```python
from build123d import *

# Parameters (mm, degrees)
IZIM2_R                     = 1
Y_KSEKLIK_EKSTR_ZYON1_DEPTH = 3


with BuildPart() as part:
    # Çizim2 → Yükseklik-Ekstrüzyon1 (new body)
    with BuildSketch(Plane(origin=(0, 0, 0), x_dir=(1, 0, 0), z_dir=(0, 1, 0))):
        with BuildLine():
            Line((2.727931774, -0.347689854), (2.491435912, -0.206753706))
            Line((2.491435912, -0.206753706), (2.246916453, -0.117755902))
            ThreePointArc((2.246916453, -0.117755902), (2.25, 0), (2.246916453, 0.117755902))
            Line((2.246916453, 0.117755902), (2.491435912, 0.206753706))
            Line((2.491435912, 0.206753706), (2.727931774, 0.347689854))
            ThreePointArc((2.727931774, 0.347689854), (2.716142937, 0.430194779), (2.701859364, 0.512304577))
            Line((2.701859364, 0.512304577), (2.433386768, 0.573261578))
            Line((2.433386768, 0.573261578), (2.173333109, 0.582342851))
            ThreePointArc((2.173333109, 0.582342851), (2.139877162, 0.695288237), (2.10055596, 0.806327886))
            Line((2.10055596, 0.806327886), (2.30560595, 0.966530497))
            Line((2.30560595, 0.966530497), (2.486975217, 1.173649979))
            ThreePointArc((2.486975217, 1.173649979), (2.450267942, 1.248473874), (2.411310133, 1.322151066))
            Line((2.411310133, 1.322151066), (2.137140773, 1.297162024))
            Line((2.137140773, 1.297162024), (1.887008778, 1.225437829))
            ThreePointArc((1.887008778, 1.225437829), (1.820288237, 1.322516818), (1.748578413, 1.41597088))
            Line((1.748578413, 1.41597088), (1.894087214, 1.631696548))
            Line((1.894087214, 1.631696548), (2.002576197, 1.884725067))
            ThreePointArc((2.002576197, 1.884725067), (1.944543648, 1.944543648), (1.884725067, 2.002576197))
            Line((1.884725067, 2.002576197), (1.631696548, 1.894087214))
            Line((1.631696548, 1.894087214), (1.41597088, 1.748578413))
            ThreePointArc((1.41597088, 1.748578413), (1.322516818, 1.820288237), (1.225437829, 1.887008778))
            Line((1.225437829, 1.887008778), (1.297162024, 2.137140773))
            Line((1.297162024, 2.137140773), (1.322151066, 2.411310133))
            ThreePointArc((1.322151066, 2.411310133), (1.248473874, 2.450267942), (1.173649979, 2.486975217))
            Line((1.173649979, 2.486975217), (0.966530497, 2.30560595))
            Line((0.966530497, 2.30560595), (0.806327886, 2.10055596))
            ThreePointArc((0.806327886, 2.10055596), (0.695288237, 2.139877162), (0.582342851, 2.173333109))
            Line((0.582342851, 2.173333109), (0.573261578, 2.433386768))
            Line((0.573261578, 2.433386768), (0.512304577, 2.701859364))
            ThreePointArc((0.512304577, 2.701859364), (0.430194779, 2.716142937), (0.347689854, 2.727931774))
            Line((0.347689854, 2.727931774), (0.206753706, 2.491435912))
            Line((0.206753706, 2.491435912), (0.117755902, 2.246916453))
            ThreePointArc((0.117755902, 2.246916453), (0, 2.25), (-0.117755902, 2.246916453))
            Line((-0.117755902, 2.246916453), (-0.206753706, 2.491435912))
            Line((-0.206753706, 2.491435912), (-0.347689854, 2.727931774))
            ThreePointArc((-0.347689854, 2.727931774), (-0.430194779, 2.716142937), (-0.512304577, 2.701859364))
            Line((-0.512304577, 2.701859364), (-0.573261578, 2.433386768))
            Line((-0.573261578, 2.433386768), (-0.582342851, 2.173333109))
            ThreePointArc((-0.582342851, 2.173333109), (-0.695288237, 2.139877162), (-0.806327886, 2.10055596))
            Line((-0.806327886, 2.10055596), (-0.966530497, 2.30560595))
            Line((-0.966530497, 2.30560595), (-1.173649979, 2.486975217))
            ThreePointArc((-1.173649979, 2.486975217), (-1.248473874, 2.450267942), (-1.322151066, 2.411310133))
            Line((-1.322151066, 2.411310133), (-1.297162024, 2.137140773))
            Line((-1.297162024, 2.137140773), (-1.225437829, 1.887008778))
            ThreePointArc((-1.225437829, 1.887008778), (-1.322516818, 1.820288237), (-1.41597088, 1.748578413))
            Line((-1.41597088, 1.748578413), (-1.631696548, 1.894087214))
            Line((-1.631696548, 1.894087214), (-1.884725067, 2.002576197))
            ThreePointArc((-1.884725067, 2.002576197), (-1.944543648, 1.944543648), (-2.002576197, 1.884725067))
            Line((-2.002576197, 1.884725067), (-1.894087214, 1.631696548))
            Line((-1.894087214, 1.631696548), (-1.748578413, 1.41597088))
            ThreePointArc((-1.748578413, 1.41597088), (-1.820288237, 1.322516818), (-1.887008778, 1.225437829))
            Line((-1.887008778, 1.225437829), (-2.137140773, 1.297162024))
            Line((-2.137140773, 1.297162024), (-2.411310133, 1.322151066))
            ThreePointArc((-2.411310133, 1.322151066), (-2.450267942, 1.248473874), (-2.486975217, 1.173649979))
            Line((-2.486975217, 1.173649979), (-2.30560595, 0.966530497))
            Line((-2.30560595, 0.966530497), (-2.10055596, 0.806327886))
            ThreePointArc((-2.10055596, 0.806327886), (-2.139877162, 0.695288237), (-2.173333109, 0.582342851))
            Line((-2.173333109, 0.582342851), (-2.433386768, 0.573261578))
            Line((-2.433386768, 0.573261578), (-2.701859364, 0.512304577))
            ThreePointArc((-2.701859364, 0.512304577), (-2.716142937, 0.430194779), (-2.727931774, 0.347689854))
            Line((-2.727931774, 0.347689854), (-2.491435912, 0.206753706))
            Line((-2.491435912, 0.206753706), (-2.246916453, 0.117755902))
            ThreePointArc((-2.246916453, 0.117755902), (-2.25, 0), (-2.246916453, -0.117755902))
            Line((-2.246916453, -0.117755902), (-2.491435912, -0.206753706))
            Line((-2.491435912, -0.206753706), (-2.727931774, -0.347689854))
            ThreePointArc((-2.727931774, -0.347689854), (-2.716142937, -0.430194779), (-2.701859364, -0.512304577))
            Line((-2.701859364, -0.512304577), (-2.433386768, -0.573261578))
            Line((-2.433386768, -0.573261578), (-2.173333109, -0.582342851))
            ThreePointArc((-2.173333109, -0.582342851), (-2.139877162, -0.695288237), (-2.10055596, -0.806327886))
            Line((-2.10055596, -0.806327886), (-2.30560595, -0.966530497))
            Line((-2.30560595, -0.966530497), (-2.486975217, -1.173649979))
            ThreePointArc((-2.486975217, -1.173649979), (-2.450267942, -1.248473874), (-2.411310133, -1.322151066))
            Line((-2.411310133, -1.322151066), (-2.137140773, -1.297162024))
            Line((-2.137140773, -1.297162024), (-1.887008778, -1.225437829))
            ThreePointArc((-1.887008778, -1.225437829), (-1.820288237, -1.322516818), (-1.748578413, -1.41597088))
            Line((-1.748578413, -1.41597088), (-1.894087214, -1.631696548))
            Line((-1.894087214, -1.631696548), (-2.002576197, -1.884725067))
            ThreePointArc((-2.002576197, -1.884725067), (-1.944543648, -1.944543648), (-1.884725067, -2.002576197))
            Line((-1.884725067, -2.002576197), (-1.631696548, -1.894087214))
            Line((-1.631696548, -1.894087214), (-1.41597088, -1.748578413))
            ThreePointArc((-1.41597088, -1.748578413), (-1.322516818, -1.820288237), (-1.225437829, -1.887008778))
            Line((-1.225437829, -1.887008778), (-1.297162024, -2.137140773))
            Line((-1.297162024, -2.137140773), (-1.322151066, -2.411310133))
            ThreePointArc((-1.322151066, -2.411310133), (-1.248473874, -2.450267942), (-1.173649979, -2.486975217))
            Line((-1.173649979, -2.486975217), (-0.966530497, -2.30560595))
            Line((-0.966530497, -2.30560595), (-0.806327886, -2.10055596))
            ThreePointArc((-0.806327886, -2.10055596), (-0.695288237, -2.139877162), (-0.582342851, -2.173333109))
            Line((-0.582342851, -2.173333109), (-0.573261578, -2.433386768))
            Line((-0.573261578, -2.433386768), (-0.512304577, -2.701859364))
            ThreePointArc((-0.512304577, -2.701859364), (-0.430194779, -2.716142937), (-0.347689854, -2.727931774))
            Line((-0.347689854, -2.727931774), (-0.206753706, -2.491435912))
            Line((-0.206753706, -2.491435912), (-0.117755902, -2.246916453))
            ThreePointArc((-0.117755902, -2.246916453), (0, -2.25), (0.117755902, -2.246916453))
            Line((0.117755902, -2.246916453), (0.206753706, -2.491435912))
            Line((0.206753706, -2.491435912), (0.347689854, -2.727931774))
            ThreePointArc((0.347689854, -2.727931774), (0.430194779, -2.716142937), (0.512304577, -2.701859364))
            Line((0.512304577, -2.701859364), (0.573261578, -2.433386768))
            Line((0.573261578, -2.433386768), (0.582342851, -2.173333109))
            ThreePointArc((0.582342851, -2.173333109), (0.695288237, -2.139877162), (0.806327886, -2.10055596))
            Line((0.806327886, -2.10055596), (0.966530497, -2.30560595))
            Line((0.966530497, -2.30560595), (1.173649979, -2.486975217))
            ThreePointArc((1.173649979, -2.486975217), (1.248473874, -2.450267942), (1.322151066, -2.411310133))
            Line((1.322151066, -2.411310133), (1.297162024, -2.137140773))
            Line((1.297162024, -2.137140773), (1.225437829, -1.887008778))
            ThreePointArc((1.225437829, -1.887008778), (1.322516818, -1.820288237), (1.41597088, -1.748578413))
            Line((1.41597088, -1.748578413), (1.631696548, -1.894087214))
            Line((1.631696548, -1.894087214), (1.884725067, -2.002576197))
            ThreePointArc((1.884725067, -2.002576197), (1.944543648, -1.944543648), (2.002576197, -1.884725067))
            Line((2.002576197, -1.884725067), (1.894087214, -1.631696548))
            Line((1.894087214, -1.631696548), (1.748578413, -1.41597088))
            ThreePointArc((1.748578413, -1.41597088), (1.820288237, -1.322516818), (1.887008778, -1.225437829))
            Line((1.887008778, -1.225437829), (2.137140773, -1.297162024))
            Line((2.137140773, -1.297162024), (2.411310133, -1.322151066))
            ThreePointArc((2.411310133, -1.322151066), (2.450267942, -1.248473874), (2.486975217, -1.173649979))
            Line((2.486975217, -1.173649979), (2.30560595, -0.966530497))
            Line((2.30560595, -0.966530497), (2.10055596, -0.806327886))
            ThreePointArc((2.10055596, -0.806327886), (2.139877162, -0.695288237), (2.173333109, -0.582342851))
            Line((2.173333109, -0.582342851), (2.433386768, -0.573261578))
            Line((2.433386768, -0.573261578), (2.701859364, -0.512304577))
            ThreePointArc((2.701859364, -0.512304577), (2.716142937, -0.430194779), (2.727931774, -0.347689854))
        make_face()
        Circle(IZIM2_R, mode=Mode.SUBTRACT)
    extrude(amount=Y_KSEKLIK_EKSTR_ZYON1_DEPTH)


solid = part.part
```
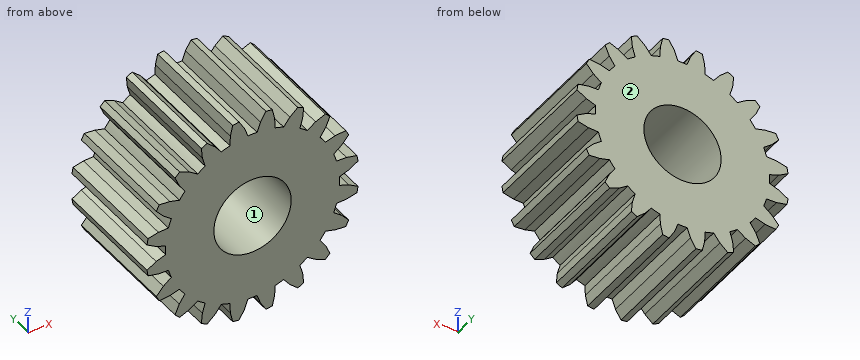
For this review, take the finished solid that the model builds, in its own axes (mm). Face numbers are marked on the shaded views. Coordinates: 2 decimals unless noted, no trailing zeros. Loops run counter-clockwise (first coordinate to the right, second up) from the corner with the lowest first, then second, coordinate; pieces in that order, holes last.
1. Mouldability with a two-part tool opening along Z and no side actions: class the marked faces 1 and 2 as +Z half, -Z half, draft (parallel to the pull), parting line (faces both ways), or undercut.
2. Insertion check: P1, Ø2.5, axis at x = 0, z = 0, coming from the +Y side. The pin has a flat end and moves straight along its axis. Give the tip position at first contact, or say it passes through.
3. Add section B-B, the plane z = 0. Give the boundary of the cut face in (x, y), then the cut area to 3 significant figures.
4. For line 1 (Z direction, x = 2.35, y = 0.3); line 2 (X direction, y = 0.5, z = 1.95); line 3 (X direction, y = 1.05, z = 2.3), list the stretches that pass through material, from the lowest coordinate up.
5. Add section A-A, the plane x = 0. Give the boundary of the cut face in (y, z).
Result:
1. face 1: undercut
1. face 2: draft
2. P1: stops at y = 3
3. outline: (-2.25, 0) - (-1, 0) - (-1, 3) - (-2.25, 3) - close; (1, 0) - (2.25, 0) - (2.25, 3) - (1, 3) - close
3. area: 7.50 mm2
4. line 1: z = -1.32 to -1.02, -0.58 to -0.16, 0.16 to 0.58, 1.02 to 1.32
4. line 2: x = -1.94 to -1.76, -1.24 to 1.24, 1.76 to 1.94
4. line 3: x = -1.31 to -0.96, -0.58 to -0.14, 0.14 to 0.58, 0.96 to 1.31
5. outline: (0, -2.25) - (3, -2.25) - (3, -1) - (0, -1) - close; (0, 1) - (3, 1) - (3, 2.25) - (0, 2.25) - close
